Work out the finished part from the listing and answer in its coordinate system (mm). Coordinates: 2 decimals unless noted, no trailing zeros. Order: outer loops, then holes, each group sorted by start corner. A loop starts at its lowest first (then second) coordinate and runs counter-clockwise, first axis right, second up. Notation, with made-up numbers: M -0.75,-24 L 53.25,-24 A23 cw 53.25,-9 Z; hole C 0,15.5 d4. An arc over 180 degrees is marked long. Answer in a Markdown table with one row per item. Add a question column.
Item 1: The part is cut by section B-B (z = 22.1). Write down the section's boundary in (x, y), then the cut area to 3 significant figures.
Item 2: The part is cut by section C-C (z = -18). Write down the section's boundary in (x, y).
Item 3: The part is cut by section A-A (y = -13.9). Write down the section's boundary in (x, z), then the cut area to 3 significant figures.
Item 4: Flat-ended cylindrical pins translate along their axes: pin 1 Ø0.9 at (x, y) = (1.5, -4) entering from +Z; pin 2 Ø1.5 at (x, y) = (1.5, -3) entering from -Z; pin 3 Ø2 at (y, z) = (13.9, -22.1) entering from +X. Find the tip coordinate at first contact, or state that the pin passes through.
Item 5: The part is cut by section D-D (x = 1.15). Write down the section's boundary in (y, z), then the cut area to 3 significant figures.
Item 6: Consider line 1 (Y direction, x = 1.5, z = 22.1); line 2 (Y direction, x = 1, z = -24); line 3 (Z direction, x = 1.35, y = 2.5). Determine where each line is inside the solid, lowest interval first. Write a range as from..to.
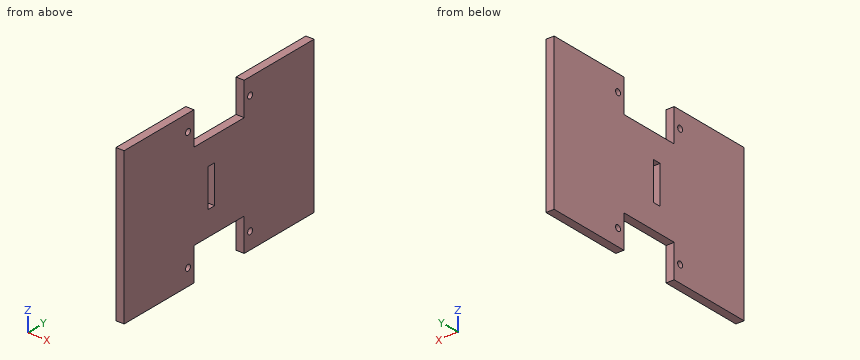
from build123d import *

# Parameters (mm, degrees)
SKETCH1_R           = 1.1
BOSS_EXTRUDE1_DEPTH = 3
SKETCH2_W           = 14
SKETCH2_H           = 3
CUT_EXTRUDE1_DEPTH  = 3


with BuildPart() as part:
    # Sketch1 → Boss-Extrude1 (new body)
    with BuildSketch(Plane(origin=(0, 0, 0), x_dir=(0, 0, -1), z_dir=(1, 0, 0))):
        Polygon((-28.2, -42.5), (28.2, -42.5), (28.2, -11.25), (16, -11.25), (16, 11.25), (28.2, 11.25), (28.2, 42.5), (-28.2, 42.5), (-28.2, 11.25), (-16, 11.25), (-16, -11.25), (-28.2, -11.25), align=None)
        with Locations((22.1, 13.9)):
            Circle(SKETCH1_R, mode=Mode.SUBTRACT)
        with Locations((22.1, -13.9)):
            Circle(SKETCH1_R, mode=Mode.SUBTRACT)
        with Locations((-22.1, -13.9)):
            Circle(SKETCH1_R, mode=Mode.SUBTRACT)
        with Locations((-22.1, 13.9)):
            Circle(SKETCH1_R, mode=Mode.SUBTRACT)
    extrude(amount=BOSS_EXTRUDE1_DEPTH)

    # Sketch2 → Cut-Extrude1 (cut)
    with BuildSketch(Plane(origin=(3, 0, 0), x_dir=(0, 0, -1), z_dir=(1, 0, 0))):
        with Locations((0, -3.45)):
            Rectangle(SKETCH2_W, SKETCH2_H)
    extrude(amount=-CUT_EXTRUDE1_DEPTH, mode=Mode.SUBTRACT)


solid = part.part
Reply:
| question | item | result |
|---|---|---|
| 1 | outline | M 0,-42.5 L 3,-42.5 L 3,-15 L 0,-15 Z; M 0,-12.8 L 3,-12.8 L 3,-11.25 L 0,-11.25 Z; M 0,11.25 L 3,11.25 L 3,12.8 L 0,12.8 Z; M 0,15 L 3,15 L 3,42.5 L 0,42.5 Z |
| 1 | area | 174 mm2 |
| 2 | outline | M 0,-42.5 L 3,-42.5 L 3,-11.25 L 0,-11.25 Z; M 0,11.25 L 3,11.25 L 3,42.5 L 0,42.5 Z |
| 3 | outline | M 0,-28.2 L 3,-28.2 L 3,-23.2 L 0,-23.2 Z; M 0,-21 L 3,-21 L 3,21 L 0,21 Z; M 0,23.2 L 3,23.2 L 3,28.2 L 0,28.2 Z |
| 3 | area | 156 mm2 |
| 4 | pin 1 | stops at z = 16 |
| 4 | pin 2 | stops at z = -16 |
| 4 | pin 3 | passes through |
| 5 | outline | M -42.5,-28.2 L -11.25,-28.2 L -11.25,-16 L 11.25,-16 L 11.25,-28.2 L 42.5,-28.2 L 42.5,28.2 L 11.25,28.2 L 11.25,16 L -11.25,16 L -11.25,28.2 L -42.5,28.2 Z; hole C -13.9,-22.1 d2.2; hole C -13.9,22.1 d2.2; hole M -4.95,-7 L -1.95,-7 L -1.95,7 L -4.95,7 Z; hole C 13.9,-22.1 d2.2; hole C 13.9,22.1 d2.2 |
| 5 | area | 4,190 mm2 |
| 6 | line 1 | y = -42.5..-15, -12.8..-11.25, 11.25..12.8, 15..42.5 |
| 6 | line 2 | y = -42.5..-11.25, 11.25..42.5 |
| 6 | line 3 | z = -16..16 |
